```python
from build123d import *

# Parameters (mm, degrees)
F1_DEPTH = 8
F2_W     = 8
F2_H     = 200
F3_DEPTH = 40
F5_DEPTH = 150


with BuildPart() as f1:
    # F0 (on Front) → F1 (new body)
    with BuildSketch(Plane.XZ):
        Polygon((0, 42), (0, 0), (98.825, 0), (98.825, 300), (48.825, 300), align=None)
        Polygon((98.825, 300), (98.825, 0), (197.65, 0), (197.65, 42), (148.825, 300), align=None)
    extrude(amount=F1_DEPTH)

    # F2 (on face) → F3 (join)
    with BuildSketch(Plane.XZ.offset(8)):
        with Locations((50.67, 100)):
            Rectangle(F2_W, F2_H)
        with Locations((146.98, 100)):
            Rectangle(F2_W, F2_H)
    extrude(amount=F3_DEPTH)

    # F4 (on face) → F5 (cut)
    with BuildSketch(Plane(origin=(46.67, 0, 0), x_dir=(0, -1, 0), z_dir=(-1, 0, 0))):
        Polygon((23, 200), (48, 50), (48, 200), align=None)
    extrude(amount=-F5_DEPTH, mode=Mode.SUBTRACT)


solid = f1.part
```
Input: part model. Units: mm. Frame: model coordinates. A direction names the side the tool comes from. Give positions to 0.01 mm unless a question says otherwise; leave off trailing zeros. Order: outer loops, then holes, each group sorted by start corner. A loop starts at its lowest first (then second) coordinate and runs counter-clockwise, first axis right, second up. Notation, with made-up numbers: (45.5, 15) - (88.5, 15) arc R25 ccw to (88.5, 52) - close; hole circle Ø9 at (-31, 88.5). An arc over 180 degrees is marked (long way). Use a Markdown table: item, result.
(1) Section query C-C (z = 86). Output: boundary loops of the cut face in (x, y).
Computed values:
| item | result |
|---|---|
| outline | (8.33, -8) - (46.67, -8) - (46.67, -42) - (54.67, -42) - (54.67, -8) - (142.98, -8) - (142.98, -42) - (150.98, -42) - (150.98, -8) - (189.32, -8) - (189.32, 0) - (8.33, 0) - close |
(2) Section query D-D (x = 106). Output: boundary loops of the cut face in (y, z), then the cut area to 3 significant figures.
Computed values:
| item | result |
|---|---|
| outline | (-8, 0) - (0, 0) - (0, 300) - (-8, 300) - close |
| area | 2,400 mm2 |
(3) Section query B-B (y = -41). Output: boundary loops of the cut face in (x, z).
Computed values:
| item | result |
|---|---|
| outline | (46.67, 0) - (54.67, 0) - (54.67, 92) - (46.67, 92) - close; (142.98, 0) - (150.98, 0) - (150.98, 92) - (142.98, 92) - close |
(4) Section query A-A (y = -13.5). Output: boundary loops of the cut face in (x, z).
Computed values:
| item | result |
|---|---|
| outline | (46.67, 0) - (54.67, 0) - (54.67, 200) - (46.67, 200) - close; (142.98, 0) - (150.98, 0) - (150.98, 200) - (142.98, 200) - close |
(5) Draft query along X for faces 4 (the flat face through (142.98, -23, 76)), 5 (the flat face through (46.67, -23, 76)), 6 (the flat face through (147, -15, 200)). Return one class per face: released by +X, released by -X, zero draft, split by the parting line, or undercut.
Computed values:
| item | result |
|---|---|
| face 4 | undercut |
| face 5 | released by -X |
| face 6 | zero draft |
(6) Line query: line 1 (X direction, y = -37.5, z = 94); line 2 (Y direction, x = 160.5, z = 79); line 3 (Y direction, x = 145, z = 180.5). Output: solid intervals per line, ascending. Write a range as from..to.
Computed values:
| item | result |
|---|---|
| line 1 | x = 46.67..54.67, 142.98..150.98 |
| line 2 | y = -8..0 |
| line 3 | y = -26.25..0 |
(7) Access query for faces 1 (the flat face through (150.98, -23, 76)), 2 (the flat face through (54.67, -23, 76)), 3 (the flat face through (51, -15, 200)). Directions: +Z, -Z, +X, -X, +Y, -Y. A direction counts if a zero-diameter tool reaches every point of the face in a straight line with its end or side. Return the directions, or none.
Computed values:
| item | result |
|---|---|
| face 1 | +Z, -Z, +X, -Y |
| face 2 | +Z, -Z, -Y |
| face 3 | +Z, +X, -X, -Y |
(8) Pin query (flat end, axial travel): pin 1 (4 mm diameter, centred on x = 47, y = -40, fed in from -Z); pin 2 (20 mm diameter, centred on y = -27.5, z = 81.5, fed in from +X); pin 3 (4 mm diameter, centred on x = 50.5, y = -12.5, fed in from +Z); pin 4 (2 mm diameter, centred on y = -33.5, z = 59.5, fed in from -X). Return the tip coordinate at first contact, or that it passes through.
Computed values:
| item | result |
|---|---|
| pin 1 | stops at z = 0 |
| pin 2 | stops at x = 150.98 |
| pin 3 | stops at z = 200 |
| pin 4 | stops at x = 46.67 |
